Can you work these out from the model? Positions are in its coordinate system, mm. A direction names the side the tool comes from. Give positions to 0.01 mm unless a question says otherwise; leave off trailing zeros. Loops run counter-clockwise (first coordinate to the right, second up) from the corner with the lowest first, then second, coordinate; pieces in that order, holes last. Notation, with made-up numbers: (-3, 72) -> (32, 72) arc R22 ccw to (32, 86) -> close; hole circle Ø7 at (74, 78.25). An arc over 180 degrees is marked (long way). Use CSV: the item, a comma, the result in double quotes.
from build123d import *

# Parameters (mm, degrees)
SKETCH2_R           = 22.5
BOSS_EXTRUDE1_DEPTH = 7
SKETCH3_R           = 18.25
BOSS_EXTRUDE2_DEPTH = 15


with BuildPart() as part:
    # Sketch2 → Boss-Extrude1 (new body)
    with BuildSketch(Plane(origin=(0, 0, 0), x_dir=(1, 0, 0), z_dir=(0, 1, 0))):
        with Locations(Location((0, 0, 0), (0, 0, 270))):
            Circle(SKETCH2_R)
    extrude(amount=BOSS_EXTRUDE1_DEPTH)

    # Sketch3 → Boss-Extrude2 (add)
    with BuildSketch(Plane(origin=(0, 7, 0), x_dir=(1, 0, 0), z_dir=(0, 1, 0))):
        with Locations(Location((0, 0, 0), (0, 0, 270))):
            Circle(SKETCH3_R)
    extrude(amount=BOSS_EXTRUDE2_DEPTH)

    # Sketch5 → CBORE for M8 Hex Head Bolt1 (revolve, cut)
    with BuildSketch(Plane(origin=(0, 0, 0), x_dir=(0, 0, -1), z_dir=(1, 0, 0))):
        Polygon((0, 0), (0, 22), (5, 22), (5, 11.68), (9.005, 11.68), (9.005, 0.025), (9.03, 0), align=None)
    revolve(axis=Axis((0, -6.35, 0), (0, 1, 0)), mode=Mode.SUBTRACT)


solid = part.part
(1) If we section it at B-B, the plane x = 0: Write out the boundary of the cut face in (y, z) (3 decimals).
Answer sheet:
outline,"(0, -22.5) -> (7, -22.5) -> (7, -18.25) -> (22, -18.25) -> (22, -5) -> (11.68, -5) -> (11.68, -9.005) -> (0.025, -9.005) -> (0, -9.03) -> close; (0, 9.03) -> (0.025, 9.005) -> (11.68, 9.005) -> (11.68, 5) -> (22, 5) -> (22, 18.25) -> (7, 18.25) -> (7, 22.5) -> (0, 22.5) -> close"
(2) Which directions (+Z, -Z, +X, -X, +Y, -Y) give clear straight access to the entire face, cutting with the end or side of a thin tool? Please do faces 5 (the face through (-4, 22, 4)), 6 (the face through (-2.7, 5.77, -8.59)).
Answer sheet:
face 5,"+Z, -Z, +X, -X, +Y"
face 6,"-Y"
(3) If we section it at A-A, the plane z = 0: Write out the boundary of the cut face in (x, y) (3 decimals), then the cut area to 3 significant figures.
Answer sheet:
outline,"(-22.5, 0) -> (-9.03, 0) -> (-9.005, 0.025) -> (-9.005, 11.68) -> (-5, 11.68) -> (-5, 22) -> (-18.25, 22) -> (-18.25, 7) -> (-22.5, 7) -> close; (5, 11.68) -> (9.005, 11.68) -> (9.005, 0.025) -> (9.03, 0) -> (22.5, 0) -> (22.5, 7) -> (18.25, 7) -> (18.25, 22) -> (5, 22) -> close"
area,"549 mm2"
(4) If I drill on L1, parallel to X at y = 16, z = 0; L2, parallel to X at y = 8, z = 0 (3 decimals); L3, parallel to Y at x = -8, z = 0, over which ranges is the centre line in solid material (lowest first)? Write a range as from..to.
Answer sheet:
L1,"x = -18.25..-5, 5..18.25"
L2,"x = -18.25..-9.005, 9.005..18.25"
L3,"y = 11.68..22"
(5) If we section it at C-C, the plane y = 17.5: Write out the boundary of the cut face in (x, z).
Answer sheet:
outline,"circle Ø36.5 at (0, 0); hole circle Ø10 at (0, 0)"
(6) If we section it at D-D, the plane z = 13.5: Write out the boundary of the cut face in (x, y), then the cut area to 3 significant figures.
Answer sheet:
outline,"(-18, 0) -> (18, 0) -> (18, 7) -> (12.28, 7) -> (12.28, 22) -> (-12.28, 22) -> (-12.28, 7) -> (-18, 7) -> close"
area,"620 mm2"
(7) Will these pins go through, and if not, where does the flat tip stop? pin 1 Ø16 at (x, z) = (0, 0) entering from +Y; pin 2 Ø4 at (x, y) = (6.5, 9.5) entering from +Z; pin 3 Ø5 at (y, z) = (16.5, 6) entering from +X; pin 4 Ø1.5 at (x, z) = (-7.5, 18) entering from +Y.
Answer sheet:
pin 1,"stops at y = 22"
pin 2,"stops at z = 17.69"
pin 3,"stops at x = 17.91"
pin 4,"stops at y = 7"
(8) We'd pull the mould along X, two halves only. Please class faces 1 (the face through (4.88, 16.77, 1.08)), 2 (the face through (18.4, 7, -0.1)), 3 (the face through (-17.816, 14.395, -3.956)), 4 (the face through (4, 11.68, 4)): released by +X, released by -X, zero draft, split by the parting line, or undercut.
Answer sheet:
face 1,"undercut"
face 2,"zero draft"
face 3,"split by the parting line"
face 4,"undercut"
